```python
from build123d import *

# Parameters (mm, degrees)
T_LE_DE_BASE_PLI_E1_DEPTH                   = 30
FRAISAGE_POUR_VIS_T_TE_FRAIS_E_M31_AT_COUNT = 2
FRAISAGE_POUR_VIS_T_TE_FRAIS_E_M31_AT_PITCH = 20
FRAISAGE_POUR_VIS_T_TE_FRAIS_E_M31_2_COUNT  = 2
FRAISAGE_POUR_VIS_T_TE_FRAIS_E_M31_2_PITCH  = 28.284271247
FRAISAGE_POUR_VIS_T_TE_FRAIS_E_M31_3_COUNT  = 2
FRAISAGE_POUR_VIS_T_TE_FRAIS_E_M31_3_PITCH  = 20
D_GAGEMENT_M41_D                            = 4.5


# Sheet-metal steps are written as plain solids
with BuildPart() as part:
    # Esquisse1 → Tôle de base pliée1 (new body)
    with BuildSketch(Plane(origin=(0, 0, 0), x_dir=(0, 0, -1), z_dir=(1, 0, 0))):
        with BuildLine():
            Line((0, 12.75), (0, 4))
            ThreePointArc((0, 4), (-1.171572875, 1.171572875), (-4, 0))
            Line((-4, 0), (-40, 0))
            Line((-40, 0), (-40, 3))
            Line((-40, 3), (-4, 3))
            ThreePointArc((-4, 3), (-3.292893219, 3.292893219), (-3, 4))
            Line((-3, 4), (-3, 12.75))
            Line((-3, 12.75), (0, 12.75))
        make_face()
    extrude(amount=T_LE_DE_BASE_PLI_E1_DEPTH)

    # Esquisse7 → Fraisage pour vis à tête fraisée M31 (revolve, cut)
    with BuildSketch(Plane(origin=(5, 3, 35), x_dir=(0, 0, 1), z_dir=(1, 0, 0))):
        Polygon((0, 0), (0, 3), (1.7, 3), (1.7, 1.45), (3.15, 0), align=None)
    fraisage_pour_vis_t_te_frais_e_m31 = revolve(axis=Axis((5, 9.35, 35), (0, -1, 0)), mode=Mode.SUBTRACT)

    # Fraisage pour vis à tête fraisée M31 at: Fraisage pour vis à tête fraisée M31 ×2
    with Locations(*[(0, 0, -i * FRAISAGE_POUR_VIS_T_TE_FRAIS_E_M31_AT_PITCH) for i in range(1, FRAISAGE_POUR_VIS_T_TE_FRAIS_E_M31_AT_COUNT)]):
        add(fraisage_pour_vis_t_te_frais_e_m31, mode=Mode.SUBTRACT)

    # Fraisage pour vis _ t_te frais_e M31 2: Fraisage pour vis à tête fraisée M31 ×2
    with Locations(*[Vector(0.7071067811865476, 0, -0.7071067811865475) * (i * FRAISAGE_POUR_VIS_T_TE_FRAIS_E_M31_2_PITCH) for i in range(1, FRAISAGE_POUR_VIS_T_TE_FRAIS_E_M31_2_COUNT)]):
        add(fraisage_pour_vis_t_te_frais_e_m31, mode=Mode.SUBTRACT)

    # Fraisage pour vis _ t_te frais_e M31 3: Fraisage pour vis à tête fraisée M31 ×2
    with Locations(*[(i * FRAISAGE_POUR_VIS_T_TE_FRAIS_E_M31_3_PITCH, 0, 0) for i in range(1, FRAISAGE_POUR_VIS_T_TE_FRAIS_E_M31_3_COUNT)]):
        add(fraisage_pour_vis_t_te_frais_e_m31, mode=Mode.SUBTRACT)

    # Dégagement M41 (through all)
    with Locations(Plane.XY.offset(3)):
        with Locations((15, 8.2)):
            Hole(D_GAGEMENT_M41_D / 2)


solid = part.part
```
Here's how the part is built. I have some questions about the finished solid (model axes, mm). A direction names the side the tool comes from. Coordinates: 2 decimals unless noted, no trailing zeros. Write each loop counter-clockwise with the first axis right and the second up, starting at its lowest first coordinate (ties: lowest second). Pieces come first, ordered by that corner, then holes. Notation, with made-up numbers: M -33,33 L -6,33 A20 ccw -6,66 Z; hole C 35,61.5 d1. An arc over 180 degrees is marked long. Answer as CSV lines item,"result". Start each with the question number.
Q1. I need wall thicknesses on probe 1 along X at (y, z) = (1.25, 35); probe 2 along Z at (x, y) = (5, 0.4); probe 3 along Z at (x, y) = (25, 0.7). Which ranges of each line are inside material? Lowest first, please. Write a range as [from, to].
Q2. For faces 4 (the cylindrical face through (23.314, 0.786, 34.779)), 5 (the flat face through (15, 11, 3)), which set-ups out of +Z, -Z, +X, -X, +Y, -Y let a thin tool reach every point of the face, with its end or its side?
Q3. Will these pins go through, and if not, where does the flat tip stop? pin 1 Ø3 at (x, z) = (25, 35) entering from +Y; pin 2 Ø1.5 at (x, z) = (3.5, 26) entering from +Y; pin 3 Ø4.5 at (x, y) = (14.5, 7) entering from +Z; pin 4 Ø4 at (x, z) = (25, 15) entering from +Y.
Q4. Suppose I cut it at D-D, the plane y = 8.2. List the corners of the cut face in (x, z) for me, then the cut area to 3 significant figures.
Q5. If we mould it in two halves opening along Z, with no side actions, what happens to faces 1 (the cylindrical face through (4.93, 0.79, 33.3)), 2 (the flat face through (0, 2.6, 15.5)), 3 (the flat face through (14.8, 5.5, 0))? For each: pulls with the +Z half, pulls with the -Z half, needs draft (parallel to the pull), parting line crosses it, or undercut.
Q6. Suppose I cut it at A-A, the plane x = 25. List the corners of the cut face in (y, z) for me, then the cut area to 3 significant figures.
Q7. Suppose I cut it at B-B, the plane x = 15. List the corners of the cut face in (y, z) for me.
Q8. Suppose I cut it at C-C, the plane z = 15. List the corners of the cut face in (x, y) for me.
Entries:
1,probe 1,"x = [0, 3.3], [6.7, 23.3], [26.7, 30]"
1,probe 2,"z = [2.26, 13.3], [16.7, 33.3], [36.7, 40]"
1,probe 3,"z = [1.74, 13.3], [16.7, 33.3], [36.7, 40]"
2,face 4,"+Y, -Y"
2,face 5,"+Z, +X, -X, +Y"
3,pin 1,"passes through"
3,pin 2,"stops at y = 3"
3,pin 3,"stops at z = 3"
3,pin 4,"stops at y = 1.85"
4,outline,"M 0,0 L 12.75,0 L 12.75,3 L 0,3 Z; M 17.25,0 L 30,0 L 30,3 L 17.25,3 Z"
4,area,"76.5 mm²"
5,face 1,"undercut"
5,face 2,"needs draft"
5,face 3,"pulls with the -Z half"
6,outline,"M 0,4 A4 ccw 4,0 L 12.75,0 L 12.75,3 L 4,3 A1 cw 3,4 L 3,11.85 L 1.55,13.3 L 0,13.3 Z; M 0,16.7 L 1.55,16.7 L 3,18.15 L 3,31.85 L 1.55,33.3 L 0,33.3 Z; M 0,36.7 L 1.55,36.7 L 3,38.15 L 3,40 L 0,40 Z"
6,area,"121 mm²"
7,outline,"M 0,4 A4 ccw 4,0 L 5.95,0 L 5.95,3 L 4,3 A1 cw 3,4 L 3,40 L 0,40 Z; M 10.45,0 L 12.75,0 L 12.75,3 L 10.45,3 Z"
8,outline,"M 0,0 L 3.3,0 L 3.3,1.55 L 1.85,3 L 0,3 Z; M 6.7,0 L 23.3,0 L 23.3,1.55 L 21.85,3 L 8.15,3 L 6.7,1.55 Z; M 26.7,0 L 30,0 L 30,3 L 28.15,3 L 26.7,1.55 Z"
